Geometry: see drawing. Coordinates: mm, zero at the bounding-box minimum. A direction names the side the tool comes from. Coordinates: 2 decimals unless noted, no trailing zeros. Loops run counter-clockwise (first coordinate to the right, second up) from the corner with the lowest first, then second, coordinate; pieces in that order, holes last. Notation, with made-up numbers: (25, -36.75) - (80, -36.75) arc R8 ccw to (80, -23.75) - close; hole circle Ø4 at (20.5, -32.75). An arc over 180 degrees is marked (long way). Use one line per item in the form item = value.
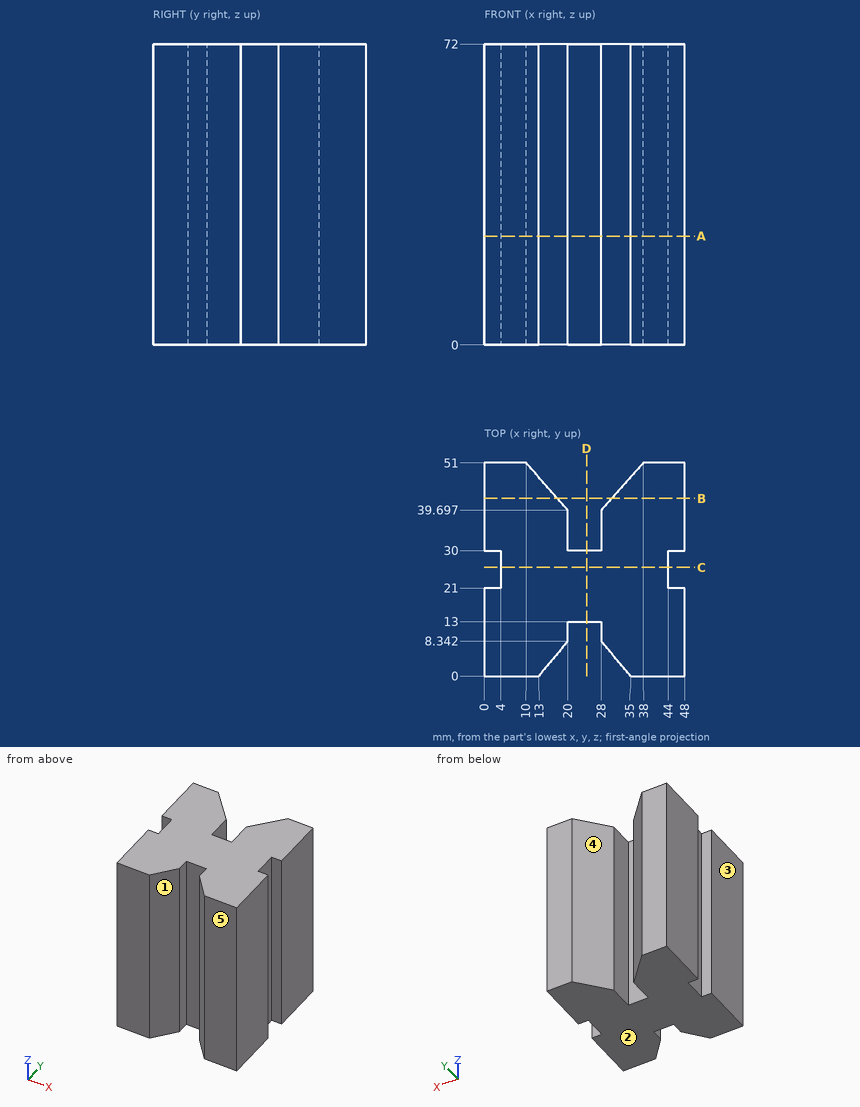
Q1. First-contact query: P1, Ø1.4, axis at y = 11.5, z = 26.5, coming from the -X side; P2, Ø2.5, axis at x = 22.5, z = 23.5, coming from the +Y side; P3, Ø1.5, axis at x = 14, z = 38, coming from the -Y side; P4, Ø9, axis at x = 22, z = 46.5, coming from the -Y side. Flat tips, straight axial feed; report the tip coordinate or a pass-through.
Check values:
P1 = 0
P2 = 30
P3 = 0.3
P4 = 5.36
Q2. Pull-direction query (X, two-part tool) for the marked faces 3, 4 and 5; classes: pulls with the +X half, pulls with the -X half, needs draft (parallel to the pull), parting line crosses it, or undercut.
Check values:
face_3 = pulls with the -X half
face_4 = undercut
face_5 = needs draft
Q3. Cut plane A-A, the plane z = 26. Return loops of the section in (x, y).
Check values:
outline = (0, 0) - (13, 0) - (20, 8.34) - (20, 13) - (28, 13) - (28, 8.34) - (35, 0) - (48, 0) - (48, 21) - (44, 21) - (44, 30) - (48, 30) - (48, 51) - (38, 51) - (28, 39.7) - (28, 30) - (20, 30) - (20, 39.7) - (10, 51) - (0, 51) - (0, 30) - (4, 30) - (4, 21) - (0, 21) - close
Q4. Cut plane C-C, the plane y = 26. Return loops of the section in (x, z).
Check values:
outline = (4, 0) - (44, 0) - (44, 72) - (4, 72) - close
Q5. Cut plane B-B, the plane y = 42.5. Return loops of the section in (x, z).
Check values:
outline = (0, 0) - (17.52, 0) - (17.52, 72) - (0, 72) - close; (30.48, 0) - (48, 0) - (48, 72) - (30.48, 72) - close
Q6. Set-up query: the marked faces 1 and 2. Return all of +Z, -Z, +X, -X, +Y, -Y with unobstructed straight access to the full face (end or side cutting, diameter ignored); none if empty.
Check values:
face_1 = +Z, -Z, -Y
face_2 = -Z, +X, -X, +Y, -Y
Q7. Cut plane D-D, the plane x = 24.5. Return loops of the section in (y, z), then the cut area to 3 significant figures.
Check values:
outline = (13, 0) - (30, 0) - (30, 72) - (13, 72) - close
area = 1,220 mm²
Q8. Ray query, line 1 along Y through (x, z) = (44.5, 10); line 2 along X through (y, z) = (10, 54); line 3 along X through (y, z) = (6, 33) (1 decimal). Return the intervals inside material, ascending. Write a range as [from, to].
Check values:
line_1 = [0, 21], [30, 51]
line_2 = [0, 20], [28, 48]
line_3 = [0, 18], [30, 48]
